Work out the finished part from the listing and answer in its coordinate system (mm). Face numbers are marked on the shaded views. A direction names the side the tool comes from. Round coordinates to 2 decimals unless told otherwise and drop trailing zeros. Write each loop counter-clockwise with the first axis right and the second up, starting at its lowest first coordinate (ties: lowest second). Pieces come first, ordered by that corner, then holes. Notation, with made-up numbers: M -10.5,48.25 L 26.5,48.25 A19 ccw 26.5,83.25 Z; hole C 8,52 d3. An arc over 180 degrees is marked long. One line per item, written item: value. Start each with the question number.
Q1. Find section B-B (x = 0). Write down the section's boundary in (y, z), and give its area (3 significant figures).
Q2. The mould has two halves that part along Z. Classify the marked faces 1, 2 and 3: released by +Z, released by -Z, zero draft, split by the parting line, or undercut.
Q3. Find section C-C (y = -3). Write down the section's boundary in (x, z).
Q4. Consider probe 1 along Z at (x, y) = (2.25, -0.5); probe 2 along Y at (x, z) = (0, -11.1); probe 3 along Y at (x, z) = (2, 4.75). Determine where each line is inside the solid, lowest interval first.
Q5. A tool of negligible diameter and unlimited length cuts with its end or side. For the marked faces 4, 5 and 6, from which of +Z, -Z, +X, -X, +Y, -Y can it reach the whole face along a straight path? Write none if from no direction.
Q6. Find section D-D (z = 1.25). Write down the section's boundary in (x, y), and give its area (3 significant figures).
Q7. Find section A-A (y = -0.75). Write down the section's boundary in (x, z), and give its area (3 significant figures).
Q8. Given pin 1 Ø1 at (x, z) = (6.5, 9.5) entering from -Y; pin 2 Ø1.4 at (x, y) = (1, -2.5) entering from +Z; pin 3 Ø3 at (y, z) = (-1.5, 0) entering from +X; pin 4 Ø2.5 at (x, y) = (0, -2.4) entering from -Z, each flat-ended and moving along its own axis, determine where each tip first touches the part or whether it passes through.
Autodesk Inventor part; units mm, degrees
ref_plane "body_to_terminal_XY" through (0, 0, 0) normal (0, -1, 0) x (1, 0, 0)
ref_plane "body_to_terminal_YZ" through (0, 0, 0) normal (1, 0, 0) x (0, 0, 1)
ref_plane "body_to_terminal_ZX" through (0, 0, 0) normal (0, 0, 1) x (0, -1, 0)
sketch "Sketch_2" plane through (0, 1.27, 0) normal (0, 1, 0) x (1, 0, 0)
  line L0 (-8.4328, -13.1318) -> (8.4328, -13.1318)
  line L1 (8.4328, -13.1318) -> (8.4328, 13.1318)
  line L2 (8.4328, 13.1318) -> (-8.4328, 13.1318)
  line L3 (-8.4328, 13.1318) -> (-8.4328, -13.1318)
extrude "Extrusion1" add sketch "Sketch_2" along normal blind 2.54
sketch "Sketch_1" plane through (0, 0, -11.2014) normal (0, 0, 1) x (1, 0, 0)
  line L0 (-2.4003, 1.27) -> (-2.4003, -3.5306)
  arc A0 (-2.4003, -3.5306) -> (2.4003, -3.5306) centre (0, -1.8973) ccw
  line L1 (2.4003, -3.5306) -> (2.4003, 1.27)
  line L2 (2.4003, 1.27) -> (-2.4003, 1.27)
  circle A1 centre (0, -2.4003) radius 1.1938
extrude "Extrusion2" add sketch "Sketch_1" along normal mid plane 0.7874
sketch "Sketch_3" plane through (0, 0, 11.2014) normal (0, 0, 1) x (1, 0, 0)
  line L0 (-2.4003, 1.27) -> (-2.4003, -3.5306)
  arc A0 (-2.4003, -3.5306) -> (2.4003, -3.5306) centre (0, -1.8973) ccw
  line L1 (2.4003, -3.5306) -> (2.4003, 1.27)
  line L2 (2.4003, 1.27) -> (-2.4003, 1.27)
  circle A1 centre (0, -2.4003) radius 1.1938
extrude "Extrusion3" add sketch "Sketch_3" along normal mid plane 0.7874
ref_plane "body_to_terminal_XY" through (0, 0, 0) normal (0, -1, 0) x (1, 0, 0)
ref_plane "body_to_terminal_YZ" through (0, 0, 0) normal (1, 0, 0) x (0, 0, 1)
ref_plane "body_to_terminal_ZX" through (0, 0, 0) normal (0, 0, 1) x (0, -1, 0)
ref_plane "wire_1_XY" through (-3.048, 0, 7.62) normal (0, 1, 0) x (1, 0, 0)
ref_plane "wire_1_YZ" through (-3.048, 0, 7.62) normal (1, 0, 0) x (0, 0, -1)
ref_plane "wire_1_ZX" through (-3.048, 0, 7.62) normal (0, 0, -1) x (0, 1, 0)
ref_plane "wire_2_XY" through (3.048, 0, 7.62) normal (0, 1, 0) x (1, 0, 0)
ref_plane "wire_2_YZ" through (3.048, 0, 7.62) normal (1, 0, 0) x (0, 0, -1)
ref_plane "wire_2_ZX" through (3.048, 0, 7.62) normal (0, 0, -1) x (0, 1, 0)
ref_plane "wire_3_XY" through (-3.048, 0, 0) normal (0, 1, 0) x (1, 0, 0)
ref_plane "wire_3_YZ" through (-3.048, 0, 0) normal (1, 0, 0) x (0, 0, -1)
ref_plane "wire_3_ZX" through (-3.048, 0, 0) normal (0, 0, -1) x (0, 1, 0)
ref_plane "wire_4_XY" through (3.048, 0, 0) normal (0, 1, 0) x (1, 0, 0)
ref_plane "wire_4_YZ" through (3.048, 0, 0) normal (1, 0, 0) x (0, 0, -1)
ref_plane "wire_4_ZX" through (3.048, 0, 0) normal (0, 0, -1) x (0, 1, 0)
ref_plane "wire_5_XY" through (-3.048, 0, -7.62) normal (0, 1, 0) x (1, 0, 0)
ref_plane "wire_5_YZ" through (-3.048, 0, -7.62) normal (1, 0, 0) x (0, 0, -1)
ref_plane "wire_5_ZX" through (-3.048, 0, -7.62) normal (0, 0, -1) x (0, 1, 0)
ref_plane "wire_6_XY" through (3.048, 0, -7.62) normal (0, 1, 0) x (1, 0, 0)
ref_plane "wire_6_YZ" through (3.048, 0, -7.62) normal (1, 0, 0) x (0, 0, -1)
ref_plane "wire_6_ZX" through (3.048, 0, -7.62) normal (0, 0, -1) x (0, 1, 0)
properties part number "WT11S_terminal"
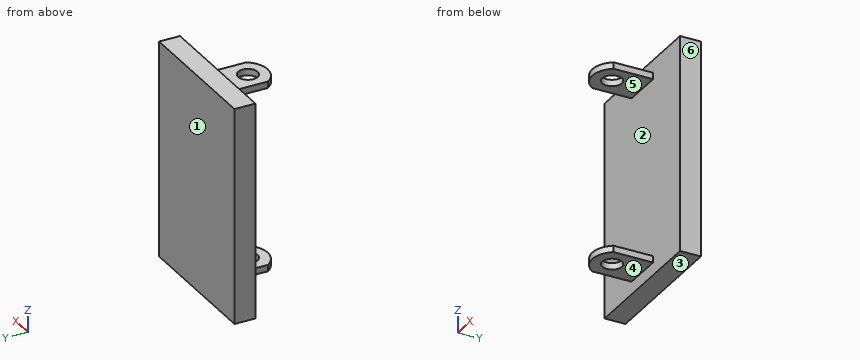
The answers:
1. outline: M -4.8,-11.6 L -3.59,-11.6 L -3.59,-10.81 L -4.8,-10.81 Z; M -4.8,10.81 L -3.59,10.81 L -3.59,11.6 L -4.8,11.6 Z; M -1.21,-11.6 L 1.27,-11.6 L 1.27,-13.13 L 3.81,-13.13 L 3.81,13.13 L 1.27,13.13 L 1.27,11.6 L -1.21,11.6 L -1.21,10.81 L 1.27,10.81 L 1.27,-10.81 L -1.21,-10.81 Z
1. area: 72.5 mm2
2. face 1: zero draft
2. face 2: undercut
2. face 3: released by -Z
3. outline: M -2.4,-11.6 L -1.03,-11.6 L -1.03,-10.81 L -2.4,-10.81 Z; M -2.4,10.81 L -1.03,10.81 L -1.03,11.6 L -2.4,11.6 Z; M 1.03,-11.6 L 2.4,-11.6 L 2.4,-10.81 L 1.03,-10.81 Z; M 1.03,10.81 L 2.4,10.81 L 2.4,11.6 L 1.03,11.6 Z
4. probe 1: -11.6 to -10.81, 10.81 to 11.6
4. probe 2: -4.8 to -3.59, -1.21 to 3.81
4. probe 3: 1.27 to 3.81
5. face 4: -Z, +X, -X, -Y
5. face 5: +X, -X, -Y
5. face 6: +Z, -Z, +X, +Y, -Y
6. outline: M -8.43,1.27 L 8.43,1.27 L 8.43,3.81 L -8.43,3.81 Z
6. area: 42.8 mm2
7. outline: M -2.4,-11.6 L 2.4,-11.6 L 2.4,-10.81 L -2.4,-10.81 Z; M -2.4,10.81 L 2.4,10.81 L 2.4,11.6 L -2.4,11.6 Z
7. area: 7.56 mm2
8. pin 1: y = 1.27
8. pin 2: z = 11.6
8. pin 3: through
8. pin 4: z = -11.6
